Model file for the job. Use its own axes, mm. A direction names the side the tool comes from. Round coordinates to 2 decimals unless told otherwise and drop trailing zeros. Loops run counter-clockwise (first coordinate to the right, second up) from the corner with the lowest first, then second, coordinate; pieces in that order, holes last. Notation, with made-up numbers: (30, -23) -> (87, -23) arc R23 ccw to (87, 16) -> close; hole circle Ø4 at (30, -6). An arc over 180 degrees is marked (long way). Use a Markdown table: item, result.
from build123d import *

# Parameters (mm, degrees)
CYLINDER049_R     = 18.5
CYLINDER049_DEPTH = 75
CYLINDER048_R     = 4
CYLINDER048_DEPTH = 350


with BuildPart() as cylinder049:
    # Cylinder049 → Cylinder049 (new body)
    with BuildSketch(Plane(origin=(336, 31, 5), x_dir=(0, 0, -1), z_dir=(1, 0, 0))):
        Circle(CYLINDER049_R)
    extrude(amount=CYLINDER049_DEPTH)


with BuildPart() as motor_threaded_bar_metal:
    # Cylinder048 → Cylinder048 (new body)
    with BuildSketch(Plane(origin=(48, 31, 12), x_dir=(0, 0, -1), z_dir=(1, 0, 0))):
        Circle(CYLINDER048_R)
    extrude(amount=CYLINDER048_DEPTH)

    # Fusion147: union Cylinder049
    add(cylinder049.part)


with BuildPart() as motor_threaded_bar_metal_1:
    # Fusion147 placement: moved
    add(motor_threaded_bar_metal.part.moved(Location((81, 0, 0))))


solid = motor_threaded_bar_metal_1.part
Q1. Drill centre lines: L1, parallel to X at y = 43, z = 18; L2, parallel to Z at x = 430.5, y = 44; L3, parallel to Y at x = 172, z = 15. Where is each one in solid material? Low to high. Write a range as from..to.
Results list:
| item | result |
|---|---|
| L1 | x = 417..492 |
| L2 | z = -8.16..18.16 |
| L3 | y = 28.35..33.65 |
Q2. Band-saw the part on A-A, the plane z = 12. Give the cut face in (x, y), plus the area to 3 significant figures.
Results list:
| item | result |
|---|---|
| outline | (129, 27) -> (417, 27) -> (417, 13.88) -> (492, 13.88) -> (492, 48.12) -> (417, 48.12) -> (417, 35) -> (129, 35) -> close |
| area | 4,870 mm² |
Q3. Tool access for faces 1 (the face through (453.98, 14.59, -3.54)), 2 (the face through (270.984, 34.966, 12.521)): list every direction of +Z, -Z, +X, -X, +Y, -Y with a clear straight run to the whole face (end or side of a thin tool).
Results list:
| item | result |
|---|---|
| face 1 | +X, -X |
| face 2 | -X |
Q4. Band-saw the part on D-D, the plane x = 164. Give the cut face in (y, z), plus the area to 3 significant figures.
Results list:
| item | result |
|---|---|
| outline | circle Ø8 at (31, 12) |
| area | 50.3 mm² |
Q5. Band-saw the part on C-C, the plane x = 448.5. Give the cut face in (y, z).
Results list:
| item | result |
|---|---|
| outline | circle Ø37 at (31, 5) |
Q6. Flat gauge pins, fed straight in: pin 1 (10 mm diameter, centred on x = 411, z = 13, fed in from +Y); pin 2 (2 mm diameter, centred on x = 244.5, y = 30.5, fed in from +Z); pin 3 (4 mm diameter, centred on y = 26, z = 4, fed in from -X). Where does each tip first touch, or does it go through?
Results list:
| item | result |
|---|---|
| pin 1 | stops at y = 35 |
| pin 2 | stops at z = 16 |
| pin 3 | stops at x = 417 |
Q7. Band-saw the part on B-B, the plane y = 31. Give the cut face in (x, z), plus the area to 3 significant figures.
Results list:
| item | result |
|---|---|
| outline | (129, 8) -> (417, 8) -> (417, -13.5) -> (492, -13.5) -> (492, 23.5) -> (417, 23.5) -> (417, 16) -> (129, 16) -> close |
| area | 5,080 mm² |
